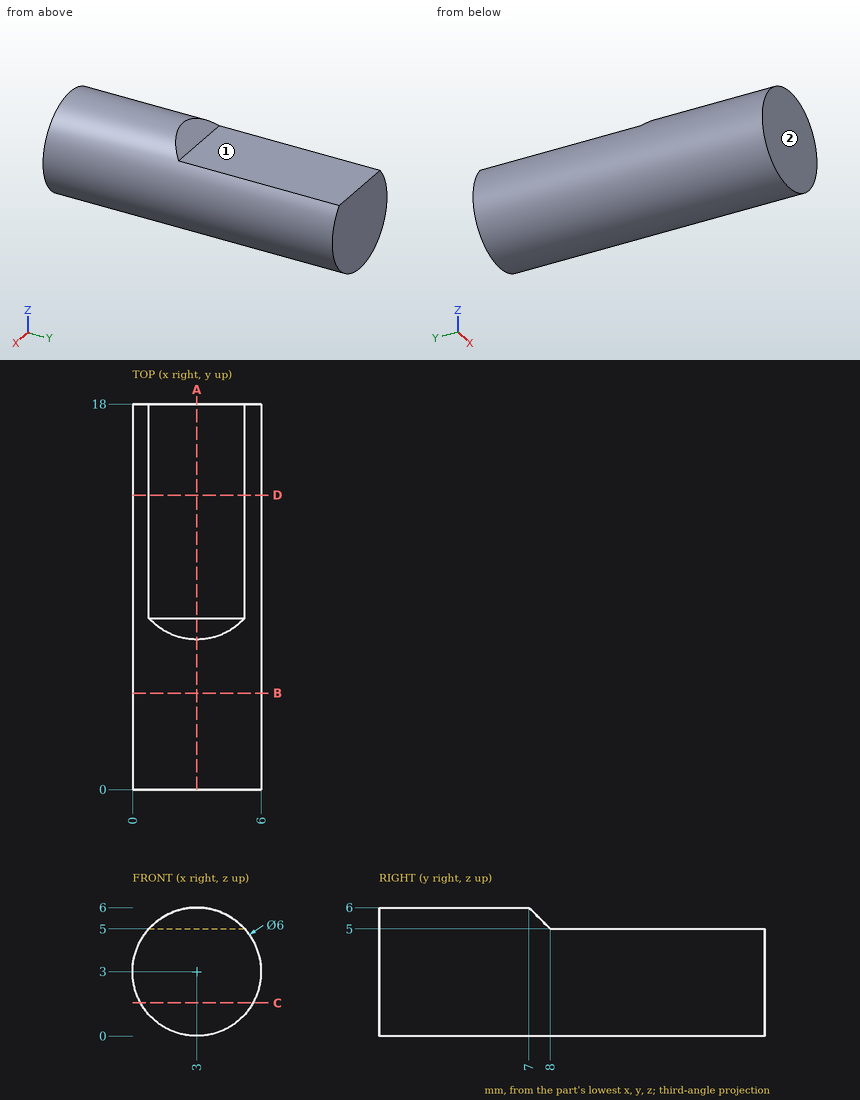
Verification items for this drawing (mm, ordinates from the low corner). A direction names the side the tool comes from. Give positions to 0.01 mm unless a question says otherwise; leave off trailing zeros. Order: outer loops, then holes, each group sorted by start corner. A loop starts at its lowest first (then second) coordinate and runs counter-clockwise, first axis right, second up.
1) Cross-section at C-C (z = 1.55). Record the boundary of the cut face in (x, y).
Results are:
outline: (0.37, 0) - (5.63, 0) - (5.63, 18) - (0.37, 18) - close
2) Material ranges on probe 1 along Z at (x, y) = (1, 8.5); probe 2 along Z at (x, y) = (3.15, 16.5); probe 3 along Y at (x, z) = (3.35, 5.3), recorded low to high.
Results are:
probe 1: z = 0.76 to 5
probe 2: z = 0 to 5
probe 3: y = 0 to 7.7
3) Cross-section at B-B (y = 4.5). Record the boundary of the cut face in (x, z).
Results are:
outline: circle Ø6 at (3, 3)
4) Cross-section at A-A (x = 3). Record the boundary of the cut face in (y, z), then the cut area to 3 significant figures.
Results are:
outline: (0, 0) - (18, 0) - (18, 5) - (8, 5) - (7, 6) - (0, 6) - close
area: 97.5 mm2
5) Tool access check on the marked faces 1 and 2. Record the directions out of +Z, -Z, +X, -X, +Y, -Y that give a thin tool (end or side, any length) a straight path to the whole face; none if there is none.
Results are:
face 1: +Z, +X, -X, +Y
face 2: +Z, -Z, +X, -X, -Y
6) Cross-section at D-D (y = 13.75). Record the boundary of the cut face in (x, z), then the cut area to 3 significant figures.
Results are:
outline: (0.76, 5) arc R3 ccw (long way) to (5.24, 5) - close
area: 25.2 mm2
7) Gauge pin test, flat ends, axial feed: pin 1 (1 mm diameter, centred on x = 5.5, y = 2, fed in from -Z); pin 2 (1 mm diameter, centred on y = 13.5, z = 1, fed in from +X). Record the tip position at first contact, or that the pin passes through.
Results are:
pin 1: stops at z = 0.76
pin 2: stops at x = 5.6
